For this review, use the dimensioned drawing (mm, ordinates from the lowest corner) and the shaded views. Give positions to 0.01 mm unless a question says otherwise; leave off trailing zeros. Order: outer loops, then holes, each group sorted by start corner. A loop starts at its lowest first (then second) coordinate and runs counter-clockwise, first axis right, second up. Notation, with made-up numbers: (3.25, 3) - (49.25, 3) arc R28 ccw to (49.25, 38) - close; hole circle Ø7 at (44.25, -5). An arc over 180 degrees is marked (long way). Use a Markdown table: item, result. Add a question column.
1) We need section A-A on x = 38. Write out the cut boundary in (y, z), then the cut area to 3 significant figures.
2) We need section B-B on z = 38. Write out the cut boundary in (x, y), then the cut area to 3 significant figures.
3) We need section C-C on y = 3. Give the number of separate pieces and of enclosed holes in the cut face, then the cut area to 3 significant figures.
4) Wall thickness on L1, parallel to X at y = 6, z = 38; L2, parallel to Z at x = 61.5, y = 3.75; L3, parallel to Z at x = 40, y = 2 (1 decimal): over which ranges is each line inside the solid? List them lowest first.
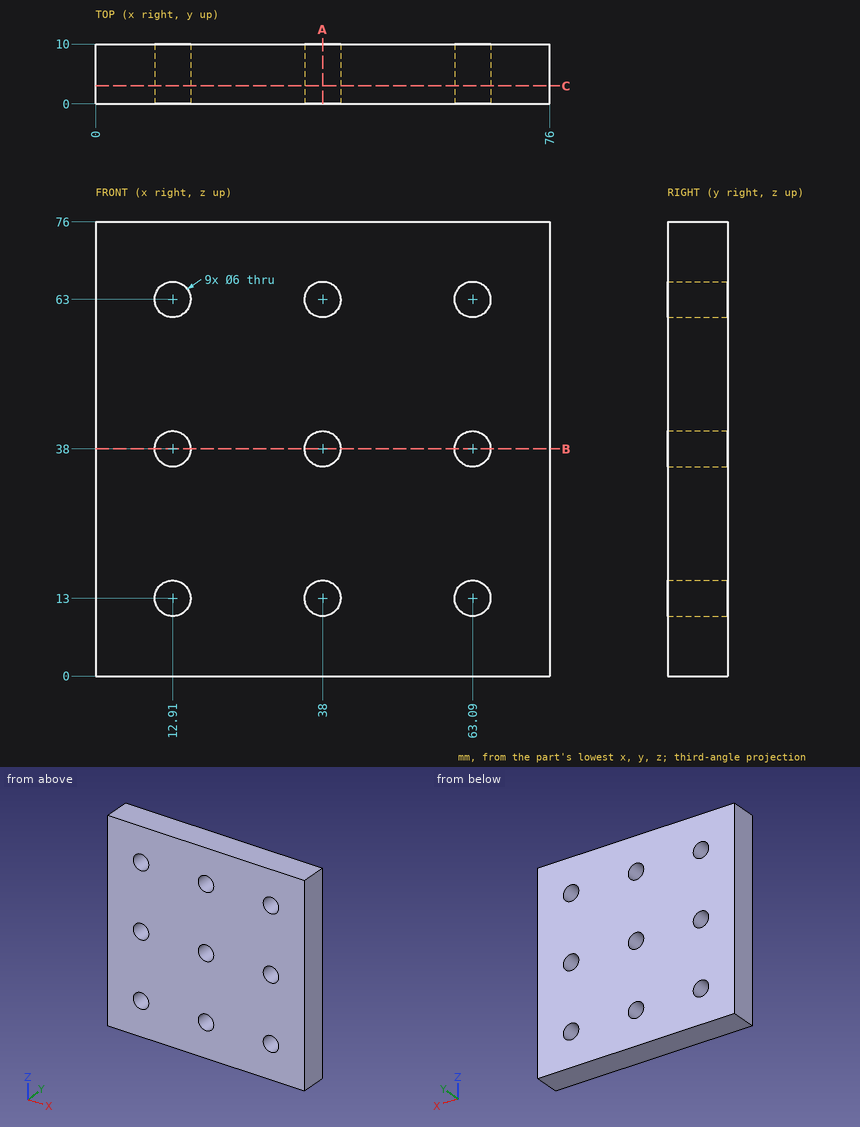
Checked values:
| question | item | result |
|---|---|---|
| 1 | outline | (0, 0) - (10, 0) - (10, 10) - (0, 10) - close; (0, 16) - (10, 16) - (10, 35) - (0, 35) - close; (0, 41) - (10, 41) - (10, 60) - (0, 60) - close; (0, 66) - (10, 66) - (10, 76) - (0, 76) - close |
| 1 | area | 580 mm² |
| 2 | outline | (0, 0) - (9.91, 0) - (9.91, 10) - (0, 10) - close; (15.91, 0) - (35, 0) - (35, 10) - (15.91, 10) - close; (41, 0) - (60.09, 0) - (60.09, 10) - (41, 10) - close; (66.09, 0) - (76, 0) - (76, 10) - (66.09, 10) - close |
| 2 | area | 580 mm² |
| 3 | separate pieces | 1 |
| 3 | enclosed holes | 9 |
| 3 | area | 5,520 mm² |
| 4 | L1 | 0 to 9.91, 15.91 to 35, 41 to 60.09, 66.09 to 76 |
| 4 | L2 | 0 to 10.46, 15.54 to 35.46, 40.54 to 60.46, 65.54 to 76 |
| 4 | L3 | 0 to 10.8, 15.2 to 35.8, 40.2 to 60.8, 65.2 to 76 |
